Part print with two shaded views. Sizes in mm from the minimum x, y, z corner. A direction names the side the tool comes from. Round coordinates to 2 decimals unless told otherwise and drop trailing zeros. Write each loop counter-clockwise with the first axis right and the second up, starting at its lowest first coordinate (ties: lowest second). Pieces come first, ordered by that corner, then holes. Notation, with made-up numbers: (0, 14.5) -> (22, 14.5) arc R8 cw to (22, 23.5) -> close; hole circle Ø2 at (-28, 30). An arc over 180 degrees is marked (long way). Put each result on its own line as item: value. Start each with the question number.
1. Saw through at B-B on y = 7.5. List the corners of the cut face in (x, z), and give its area (3 significant figures).
2. 3-axis set-ups, long thin cutter, end or side, ignore diameter. For the marked faces 4 and 5: which of +Z, -Z, +X, -X, +Y, -Y reach the whole face in a straight line?
3. Pull direction Z, two halves, no side cores. Call the marked faces 1, 2 and 3: pulls with the +Z half, pulls with the -Z half, needs draft (parallel to the pull), parting line crosses it, or undercut.
4. Flat gauge pins, fed straight in: P1, Ø6.5, axis at y = 9, z = 10, coming from the +X side; P2, Ø1, axis at x = 17.5, y = 13, coming from the -Z side. Where does each tip first touch, or does it go through?
5. Saw through at A-A on x = 10. List the corners of the cut face in (y, z).
6. Saw through at C-C on z = 10. List the corners of the cut face in (x, y).
7. Drill centre lines: line 1 (Y direction, x = 0.9, z = 10); line 2 (X direction, y = 16.5, z = 4); line 3 (Z direction, x = 6.5, y = 10.75). Where is each one in solid material? Low to high. Write a range as from..to.
8. Saw through at D-D on y = 3.5. List the corners of the cut face in (x, z), and give its area (3 significant figures).
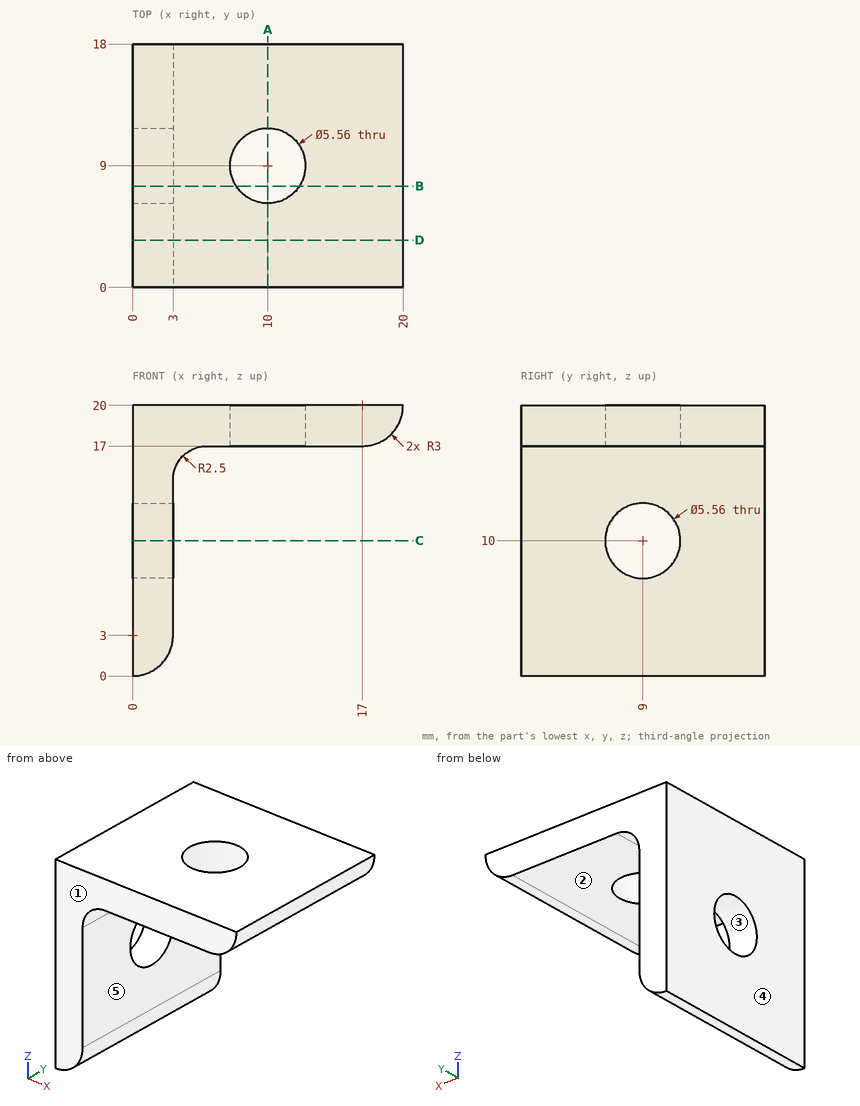
Return value:
1. outline: (0, 0) arc R3 ccw to (3, 3) -> (3, 7.66) -> (0, 7.66) -> close; (0, 12.34) -> (3, 12.34) -> (3, 14.5) arc R2.5 cw to (5.5, 17) -> (7.66, 17) -> (7.66, 20) -> (0, 20) -> close; (12.34, 17) -> (17, 17) arc R3 ccw to (20, 20) -> (12.34, 20) -> close
1. area: 80.4 mm^2
2. face 4: +Z, -Z, -X, +Y, -Y
2. face 5: -Z, +X, +Y, -Y
3. face 1: needs draft
3. face 2: pulls with the -Z half
3. face 3: undercut
4. P1: stops at x = 3
4. P2: stops at z = 17
5. outline: (0, 17) -> (6.22, 17) -> (6.22, 20) -> (0, 20) -> close; (11.78, 17) -> (18, 17) -> (18, 20) -> (11.78, 20) -> close
6. outline: (0, 0) -> (3, 0) -> (3, 6.22) -> (0, 6.22) -> close; (0, 11.78) -> (3, 11.78) -> (3, 18) -> (0, 18) -> close
7. line 1: y = 0..6.22, 11.78..18
7. line 2: x = 0..3
7. line 3: z = 17..20
8. outline: (0, 0) arc R3 ccw to (3, 3) -> (3, 14.5) arc R2.5 cw to (5.5, 17) -> (17, 17) arc R3 ccw to (20, 20) -> (0, 20) -> close
8. area: 108 mm^2
